Can you work these out from the model? Positions are in its coordinate system, mm. A direction names the side the tool comes from. Give positions to 0.01 mm unless a question says otherwise; leave off trailing zeros. Loops run counter-clockwise (first coordinate to the right, second up) from the corner with the lowest first, then second, coordinate; pieces in that order, holes last. Notation, with made-up numbers: (25.25, 26) - (43.25, 26) arc R18 ccw to (43.25, 32) - close; hole circle Ø7 at (-21, 25.5). An arc over 180 degrees is marked (long way). Answer in a Markdown table with one row per item.
from build123d import *

# Parameters (mm, degrees)
F1_DEPTH  = 20
F3_DEPTH  = 20.001
F4_W      = 20
F4_H      = 20
F5_DEPTH  = 3
F6_W      = 20
F6_H      = 3
F7_DEPTH  = 30
F8_R      = 2.5
F9_DEPTH  = 3.001
F10_W     = 20
F10_H     = 20
F11_DEPTH = 3
F12_W     = 20
F12_H     = 3
F13_DEPTH = 30
F14_R     = 2.5
F15_DEPTH = 3.001
F16_W     = 20
F16_H     = 20
F17_DEPTH = 3
F18_W     = 20
F18_H     = 3
F19_DEPTH = 30
F20_R     = 2.5
F21_DEPTH = 3.001


with BuildPart() as f1:
    # F0 (on Top) → F1 (new body)
    with BuildSketch(Plane.XY):
        Polygon((0, 0), (150, 0), (75, 129.9038105677), align=None)
    extrude(amount=F1_DEPTH)

    # F2 (on face) → F3 (cut, through all)
    with BuildSketch(Plane.XY.offset(20)):
        Polygon((75, 129.9038105677), (65, 112.583302492), (85, 112.583302492), align=None)
        Polygon((20, 0), (10, 17.3205080757), (0, 0), align=None)
        Polygon((140, 17.3205080757), (130, 0), (150, 0), align=None)
    extrude(amount=-F3_DEPTH, mode=Mode.SUBTRACT)

    # F4 (on face) → F5 (join)
    with BuildSketch(Plane(origin=(97.5, -56.291651246, 0), x_dir=(0.5, 0.8660254038, 0), z_dir=(0.8660254038, -0.5, 0))):
        with Locations((75, -10)):
            Rectangle(F4_W, F4_H)
        with Locations((75, 10)):
            Rectangle(F4_W, F4_H)
    extrude(amount=F5_DEPTH)

    # F6 (on face) → F7 (join)
    with BuildSketch(Plane(origin=(100.0980762114, -57.791651246, 0), x_dir=(0.5, 0.8660254038, 0), z_dir=(0.8660254038, -0.5, 0))):
        with Locations((75, -18.5)):
            Rectangle(F6_W, F6_H)
    extrude(amount=F7_DEPTH)

    # F8 (on face) → F9 (cut, through all)
    with BuildSketch(Plane.XY.offset(-17)):
        with Locations((150.5884572681, -0.3397459622)):
            Circle(F8_R)
    extrude(amount=-F9_DEPTH, mode=Mode.SUBTRACT)

    # F10 (on face) → F11 (join)
    with BuildSketch(Plane(origin=(0, 112.583302492, 0), x_dir=(-1, 0, 0), z_dir=(0, 1, 0))):
        with Locations((-75, 10)):
            Rectangle(F10_W, F10_H)
        with Locations((-75, -10)):
            Rectangle(F10_W, F10_H)
    extrude(amount=F11_DEPTH)

    # F12 (on face) → F13 (join)
    with BuildSketch(Plane(origin=(0, 115.583302492, 0), x_dir=(-1, 0, 0), z_dir=(0, 1, 0))):
        with Locations((-75, -18.5)):
            Rectangle(F12_W, F12_H)
    extrude(amount=F13_DEPTH)

    # F14 (on face) → F15 (cut, through all)
    with BuildSketch(Plane.XY.offset(-17)):
        with Locations((75, 130.583302492)):
            Circle(F14_R)
    extrude(amount=-F15_DEPTH, mode=Mode.SUBTRACT)

    # F16 (on face) → F17 (join)
    with BuildSketch(Plane(origin=(15, 8.6602540378, 0), x_dir=(0.5, -0.8660254038, 0), z_dir=(-0.8660254038, -0.5, 0))):
        with Locations((0, -10)):
            Rectangle(F16_W, F16_H)
        with Locations((0, 10)):
            Rectangle(F16_W, F16_H)
    extrude(amount=F17_DEPTH)

    # F18 (on face) → F19 (join)
    with BuildSketch(Plane(origin=(12.4019237886, 7.1602540378, 0), x_dir=(0.5, -0.8660254038, 0), z_dir=(-0.8660254038, -0.5, 0))):
        with Locations((0, -18.5)):
            Rectangle(F18_W, F18_H)
    extrude(amount=F19_DEPTH)

    # F20 (on face) → F21 (cut, through all)
    with BuildSketch(Plane.XY.offset(-17)):
        with Locations((-0.5884572681, -0.3397459622)):
            Circle(F20_R)
    extrude(amount=-F21_DEPTH, mode=Mode.SUBTRACT)


solid = f1.part
Q1. Imagine slicing it at D-D, the plane y = 100.5. Write out the boundary of the cut face in (x, z).
Checked values:
| item | result |
|---|---|
| outline | (58.02, 0) - (91.98, 0) - (91.98, 20) - (58.02, 20) - close |
Q2. If we mould it in two halves opening along X, with no side actions, what happens to faces 1 (the face through (112.88, 64.29, 9.86)), 2 (the face through (-3, -2, -17)), 3 (the face through (14.93, 8.78, -9.86))? For each: released by +X, released by -X, zero draft, split by the parting line, or undercut.
Checked values:
| item | result |
|---|---|
| face 1 | released by +X |
| face 2 | zero draft |
| face 3 | undercut |
Q3. Imagine slicing it at A-A, the plane x = 75. Write out the boundary of the cut face in (y, z), and give its area (3 significant figures).
Checked values:
| item | result |
|---|---|
| outline | (0, 0) - (112.58, 0) - (112.58, -20) - (128.08, -20) - (128.08, -17) - (115.58, -17) - (115.58, 20) - (0, 20) - close; (133.08, -20) - (145.58, -20) - (145.58, -17) - (133.08, -17) - close |
| area | 2,450 mm² |
Q4. On a 3-axis mill with a long thin cutter (end or side, diameter ignored), from which of +Z, -Z, +X, -X, +Y, -Y can I reach the whole of each face in a straight line? I mean faces 4 (the face through (75, 112.583, -10)), 5 (the face through (147, 1, -17)), 6 (the face through (134.93, 8.54, -9.86)), 7 (the face through (131.521, -0.878, -7.501)). Say none if no direction works.
Checked values:
| item | result |
|---|---|
| face 4 | -Z, +X, -X, -Y |
| face 5 | +Z, +X, -Y |
| face 6 | -Z, +Y |
| face 7 | +Z, -Z, -Y |
Q5. If I drill on line 1 (Y direction, x = 75, z = -18.9); line 2 (Y direction, x = 79.5, z = 6.5); line 3 (Z direction, x = 84, y = 85.5), over which ranges is the centre line in solid material (lowest first)? Write a range as [from, to].
Checked values:
| item | result |
|---|---|
| line 1 | y = [112.58, 128.08], [133.08, 145.58] |
| line 2 | y = [0, 115.58] |
| line 3 | z = [0, 20] |
Q6. Imagine slicing it at C-C, the plane z = 14.5. Write out the boundary of the cut face in (x, y).
Checked values:
| item | result |
|---|---|
| outline | (7.4, 15.82) - (17.4, -1.5) - (20, 0) - (130, 0) - (132.6, -1.5) - (142.6, 15.82) - (140, 17.32) - (85, 112.58) - (85, 115.58) - (65, 115.58) - (65, 112.58) - (10, 17.32) - close |
Q7. Imagine slicing it at B-B, the plane z = -13. Write out the boundary of the cut face in (x, y).
Checked values:
| item | result |
|---|---|
| outline | (7.4, 15.82) - (17.4, -1.5) - (20, 0) - (10, 17.32) - close; (65, 112.58) - (85, 112.58) - (85, 115.58) - (65, 115.58) - close; (130, 0) - (132.6, -1.5) - (142.6, 15.82) - (140, 17.32) - close |
Q8. For pin 1 (1.5 mm diameter, centred on x = 17, z = 10.5, fed in from -Y); pin 2 (22 mm diameter, centred on x = 74.5, z = 10, fed in from +Y); pin 3 (2 mm diameter, centred on y = 2.5, z = 7, fed in from -X); pin 4 (4.5 mm diameter, centred on x = -0.59, y = -0.34, fed in from -Z), each with a flat end and sliding along its axis, tell me the tip position at first contact or that it passes through.
Checked values:
| item | result |
|---|---|
| pin 1 | stops at y = -1.5 |
| pin 2 | stops at y = 115.58 |
| pin 3 | stops at x = 14.52 |
| pin 4 | passes through |
